Geometry check sheet. Reference: the model listing, model coordinates, mm. Face numbers are marked on the shaded views. Round coordinates to 2 decimals unless told otherwise and drop trailing zeros. Order: outer loops, then holes, each group sorted by start corner. A loop starts at its lowest first (then second) coordinate and runs counter-clockwise, first axis right, second up.
```python
from build123d import *

# Parameters (mm, degrees)
EXTRUDE_1_DEPTH                 = 10
SKETCH_4_W                      = 7.875
SKETCH_4_H                      = 20
EXTRUDE_2_DEPTH                 = 40
CUT_EXTRUDE_1_REACH             = 116.35
SKETCH_5_R                      = 2.15
CUT_EXTRUDE_1_DIRECTION_2_DEPTH = 53
CUT_EXTRUDE_2_REACH             = 107.272
SKETCH_6_R                      = 2.15
FILLET_1_R                      = 5
FILLET_2_R                      = 5
SKETCH_7_W                      = 7.875
SKETCH_7_H                      = 20
EXTRUDE_3_DEPTH                 = 18
CUT_EXTRUDE_3_REACH             = 116.35
SKETCH_8_R                      = 2.15
EXTRUDE_8_DEPTH                 = 20
SKETCH_15_W                     = 52.625
SKETCH_15_H                     = 20
EXTRUDE_9_DEPTH                 = 40
CUT_EXTRUDE_START               = -7.875
SKETCH_14_R                     = 3.5
CUT_EXTRUDE_8_DEPTH             = 54
CUT_EXTRUDE_10_DEPTH            = 20


with BuildPart() as part:
    # 草图1 → 凸台-拉伸1 (new body)
    with BuildSketch(Plane(origin=(0, 0, 0), x_dir=(1, 0, 0), z_dir=(0, 1, 0))):
        Polygon((5.931150433, 81.572237736), (53.180774799, 81.572237736), (53.180774799, 61.572237736), (42.680774799, 42.721022935), (42.680774799, 31.757290204), (42.680774799, -57.600660719), (42.680774799, -67.427762264), (0.431150433, -67.427762264), (-17.319225201, -67.427762264), (-17.319225201, 81.572237736), align=None)
        Polygon((47.930774799, 61.572237736), (42.680774799, 61.572237736), (42.680774799, 52.689495612), align=None, mode=Mode.SUBTRACT)
        Polygon((25.906315323, 61.572237736), (-7.319225201, 61.572237736), (-7.319225201, -49.220735683), align=None, mode=Mode.SUBTRACT)
        Polygon((0.431150433, -52.427762264), (32.680774799, -52.427762264), (32.680774799, 56.508121895), align=None, mode=Mode.SUBTRACT)
    extrude(amount=EXTRUDE_1_DEPTH)

    # 草图4 → 凸台-拉伸2 (add)
    with BuildSketch(Plane(origin=(0, 10, 0), x_dir=(1, 0, 0), z_dir=(0, 1, 0))):
        with Locations((49.243274799, 71.572237736)):
            Rectangle(SKETCH_4_W, SKETCH_4_H)
    extrude(amount=EXTRUDE_2_DEPTH)

    # 草图5 → 切除-拉伸1 (cut, up to next)
    with BuildSketch(Plane.ZY.offset(-45.305774799), mode=Mode.PRIVATE) as cut_extrude_1_sk1:
        with Locations(Location((-75.572237736, 14.7, 0), (0, 0, 180))):
            Circle(SKETCH_5_R)
    cut_extrude_1_tool1 = extrude(cut_extrude_1_sk1.sketch, amount=-CUT_EXTRUDE_1_REACH, mode=Mode.PRIVATE) & part.part
    # 草图5 → 切除-拉伸1 (cut, up to next)
    with BuildSketch(Plane.ZY.offset(-45.305774799), mode=Mode.PRIVATE) as cut_extrude_1_sk2:
        with Locations(Location((-67.572237736, 14.7, 0), (0, 0, 180))):
            Circle(SKETCH_5_R)
    cut_extrude_1_tool2 = extrude(cut_extrude_1_sk2.sketch, amount=-CUT_EXTRUDE_1_REACH, mode=Mode.PRIVATE) & part.part
    # 草图5 → 切除-拉伸1 (cut, up to next)
    with BuildSketch(Plane.ZY.offset(-45.305774799), mode=Mode.PRIVATE) as cut_extrude_1_sk3:
        with Locations(Location((-71.572237736, 40.7, 0), (0, 0, 180))):
            Circle(SKETCH_5_R)
    cut_extrude_1_tool3 = extrude(cut_extrude_1_sk3.sketch, amount=-CUT_EXTRUDE_1_REACH, mode=Mode.PRIVATE) & part.part
    add(cut_extrude_1_tool1.solids().sort_by_distance((45.305775, 14.7, -75.572238))[0], mode=Mode.SUBTRACT)
    add(cut_extrude_1_tool2.solids().sort_by_distance((45.305775, 14.7, -67.572238))[0], mode=Mode.SUBTRACT)
    add(cut_extrude_1_tool3.solids().sort_by_distance((45.305775, 40.7, -71.572238))[0], mode=Mode.SUBTRACT)

    # 草图5 → 切除-拉伸1 direction 2 (cut)
    with BuildSketch(Plane.ZY.offset(-45.305774799)):
        with Locations(Location((-75.572237736, 14.7, 0), (0, 0, 180))):
            Circle(SKETCH_5_R)
        with Locations(Location((-67.572237736, 14.7, 0), (0, 0, 180))):
            Circle(SKETCH_5_R)
        with Locations(Location((-71.572237736, 40.7, 0), (0, 0, 180))):
            Circle(SKETCH_5_R)
    extrude(amount=CUT_EXTRUDE_1_DIRECTION_2_DEPTH, mode=Mode.SUBTRACT)

    # 草图6 → 切除-拉伸2 (cut, up to next)
    with BuildSketch(Plane(origin=(0, 10, 0), x_dir=(1, 0, 0), z_dir=(0, 1, 0)), mode=Mode.PRIVATE) as cut_extrude_2_sk1:
        with Locations(Location((-8.019225201, -61.542634482, 0), (0, 0, 270))):
            Circle(SKETCH_6_R)
    cut_extrude_2_tool1 = extrude(cut_extrude_2_sk1.sketch, amount=-CUT_EXTRUDE_2_REACH, mode=Mode.PRIVATE) & part.part
    # 草图6 → 切除-拉伸2 (cut, up to next)
    with BuildSketch(Plane(origin=(0, 10, 0), x_dir=(1, 0, 0), z_dir=(0, 1, 0)), mode=Mode.PRIVATE) as cut_extrude_2_sk2:
        with Locations(Location((32.680774799, -58.742634482, 0), (0, 0, 270))):
            Circle(SKETCH_6_R)
    cut_extrude_2_tool2 = extrude(cut_extrude_2_sk2.sketch, amount=-CUT_EXTRUDE_2_REACH, mode=Mode.PRIVATE) & part.part
    add(cut_extrude_2_tool1.solids().sort_by_distance((-8.019225, 10, 61.542634))[0], mode=Mode.SUBTRACT)
    add(cut_extrude_2_tool2.solids().sort_by_distance((32.680775, 10, 58.742634))[0], mode=Mode.SUBTRACT)

    # 圆角1
    fillet_1_edges = [part.edges().sort_by_distance(p)[0] for p in [
        (-17.319225201, 5, 67.427762264),
        (-17.319225201, 5, -81.572237736),
        (42.680774799, 5, 67.427762264),
    ]]
    fillet(fillet_1_edges, radius=FILLET_1_R)

    # 圆角2
    fillet_2_edges = [part.edges().sort_by_distance(p)[0] for p in [
        (32.680774799, 5, 52.427762264),
    ]]
    fillet(fillet_2_edges, radius=FILLET_2_R)

    # 草图7 → 凸台-拉伸3 (add)
    with BuildSketch(Plane.XZ):
        with Locations((49.243274799, -71.572237736)):
            Rectangle(SKETCH_7_W, SKETCH_7_H)
    extrude(amount=EXTRUDE_3_DEPTH)

    # 草图8 → 切除-拉伸3 (cut, up to next)
    with BuildSketch(Plane.ZY.offset(-45.305774799), mode=Mode.PRIVATE) as cut_extrude_3_sk1:
        with Locations((-71.572237736, -11.3)):
            Circle(SKETCH_8_R)
    cut_extrude_3_tool1 = extrude(cut_extrude_3_sk1.sketch, amount=-CUT_EXTRUDE_3_REACH, mode=Mode.PRIVATE) & part.part
    add(cut_extrude_3_tool1.solids().sort_by_distance((45.305775, -11.3, -71.572238))[0], mode=Mode.SUBTRACT)

    # 草图13 → 凸台-拉伸8 (add)
    with BuildSketch(Plane.XY.offset(-61.572237736)):
        Polygon((45.305774799, 0), (45.305774799, -18), (-7.319225201, 0), align=None)
    extrude(amount=-EXTRUDE_8_DEPTH)

    # 草图15 → 凸台-拉伸9 (add)
    with BuildSketch(Plane(origin=(0, 10, 0), x_dir=(1, 0, 0), z_dir=(0, 1, 0))):
        with Locations((18.993274799, 71.572237736)):
            Rectangle(SKETCH_15_W, SKETCH_15_H)
    extrude(amount=EXTRUDE_9_DEPTH)

    # 草图14 → 切除-拉伸8 (cut)
    with BuildSketch(Plane(origin=(53.180774799, 0, 0), x_dir=(0, 0, -1), z_dir=(1, 0, 0)).offset(CUT_EXTRUDE_START)):
        with Locations((71.572237736, 40.7)):
            Circle(SKETCH_14_R)
        with Locations((67.572237736, 14.7)):
            Circle(SKETCH_14_R)
        with Locations((75.572237736, 14.7)):
            Circle(SKETCH_14_R)
        with Locations((71.572237736, -11.3)):
            Circle(SKETCH_14_R)
    extrude(amount=-CUT_EXTRUDE_8_DEPTH, mode=Mode.SUBTRACT)

    # 草图17 → 切除-拉伸10 (cut)
    with BuildSketch(Plane.XY.offset(-61.572237736)):
        Polygon((-7.319225201, 10), (-7.319225201, 50), (45.305774799, 50), align=None)
    extrude(amount=-CUT_EXTRUDE_10_DEPTH, mode=Mode.SUBTRACT)


solid = part.part
```
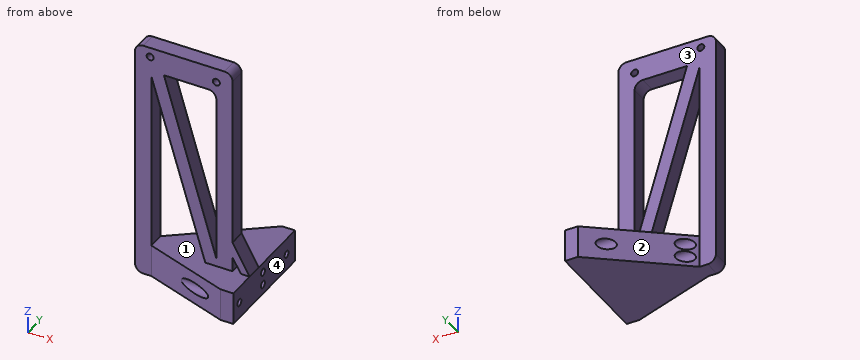
(1) Material ranges on line 1 (Z direction, x = 47.5, y = 14.7); line 2 (Z direction, x = 18.5, y = 14.7); line 3 (X direction, y = 9.5, z = -9), recorded low to high.
Returned:
line 1: z = -81.57 to -77.72, -73.42 to -69.72, -65.42 to -61.57
line 2: z = -81.57 to -79.07, -72.07 to -71.07, -64.07 to -61.57
line 3: x = -17.32 to -7.32, 10.14 to 18.62, 32.68 to 42.68
(2) Sectioned sample at A-A, the plane x = 20.5. Record the cut outline in (y, z).
Returned:
outline: (-9.52, -81.57) - (31.15, -81.57) - (31.15, -61.57) - (-9.52, -61.57) - (-9.52, -68.56) arc R3.5 cw to (-9.52, -74.58) - close; (0, -43.54) - (10, -43.54) - (10, -15.36) - (0, -15.36) - close; (0, 52.43) - (10, 52.43) - (10, 67.43) - (0, 67.43) - close; hole circle Ø7 at (14.7, -75.57); hole circle Ø7 at (14.7, -67.57)
(3) Sectioned sample at D-D, the plane y = 8. Record the cut outline in (x, z).
Returned:
outline: (-17.32, -76.57) arc R5 ccw to (-12.32, -81.57) - (53.18, -81.57) - (53.18, -61.57) - (42.68, -42.72) - (42.68, 62.43) arc R5 ccw to (37.68, 67.43) - (-12.32, 67.43) arc R5 ccw to (-17.32, 62.43) - close; hole circle Ø4.3 at (-8.02, 61.54); hole (-7.32, -61.57) - (25.91, -61.57) - (-7.32, 49.22) - close; hole (0.43, 52.43) - (32.68, -56.51) - (32.68, 47.43) arc R5 ccw to (27.68, 52.43) - close; hole circle Ø4.3 at (32.68, 58.74); hole (42.68, -61.57) - (47.93, -61.57) - (42.68, -52.69) - close
(4) Depth check by flat-ended pin: P1, Ø6.5, axis at y = 14.7, z = -75.57, coming from the -X side; P2, Ø5, axis at x = 32.68, z = 58.74, coming from the -Y side; P3, Ø12, axis at x = 15, z = -63, coming from the -Y side. Enter the tip coordinate at first touch or a pass-through.
Returned:
P1: stops at x = 45.31
P2: stops at y = 0
P3: stops at y = -9.69
(5) Draft check along X on the marked faces 1, 2, 3 and 4. Enter one of: released by +X, released by -X, zero draft, split by the parting line, or undercut.
Returned:
face 1: undercut
face 2: released by -X
face 3: zero draft
face 4: released by +X
(6) Sectioned sample at C-C, the plane z = -22. Record the cut outline in (x, y), and give its area (3 significant figures).
Returned:
outline: (-17.32, 0) - (-7.32, 0) - (-7.32, 10) - (-17.32, 10) - close; (14.04, 0) - (22.46, 0) - (22.46, 10) - (14.04, 10) - close; (32.68, 0) - (42.68, 0) - (42.68, 10) - (32.68, 10) - close
area: 284 mm2
(7) Sectioned sample at B-B, the plane y = 40.7. Record the cut outline in (x, z).
Returned:
outline: (33.07, -81.57) - (53.18, -81.57) - (53.18, -73.72) - (45.31, -73.72) - (45.31, -75.07) - (33.07, -75.07) - close; (33.07, -68.07) - (45.31, -68.07) - (45.31, -69.42) - (53.18, -69.42) - (53.18, -61.57) - (33.07, -61.57) - close
